Autodesk Inventor part; units mm, degrees
ref_plane "YZ Plane" through (0, 0, 0) normal (1, 0, 0) x (0, 1, 0)
ref_plane "XZ Plane" through (0, 0, 0) normal (0, 1, 0) x (-1, 0, 0)
ref_plane "XY Plane" through (0, 0, 0) normal (0, 0, 1) x (1, 0, 0)
sketch "Esquisse1" plane through (0, 0, 0) normal (0, 0, 1) x (1, 0, 0)
  line L0 (0, -2.6) -> (0, 15.6)
  line L1 (-12.6, 0) -> (5.6, 0)
  line L2 (-10, 10) -> (0, 10)
  line L3 (0, 10) -> (0, 0)
  line L4 (0, 0) -> (-10, 0)
  line L5 (-10, 0) -> (-10, 10)
  line L6 (-10, 10) -> (0, 10)
  line L7 (0, 10) -> (0, 13)
  line L8 (0, 13) -> (-10, 13)
  line L9 (-10, 13) -> (-10, 10)
  line L10 (0, 0) -> (3, 0)
  line L11 (3, 0) -> (3, 13)
  line L12 (3, 13) -> (0, 13)
  line L13 (0, 13) -> (0, 0)
  dimension "d0" = 10
  dimension "d1" = 10
  dimension "d2" = 3
  dimension "d3" = 3
extrude "Extrusion1" add sketch "Esquisse1" along normal blind 2
sketch "Esquisse2" plane through (0, 0, 2) normal (0, 0, 1) x (1, 0, 0)
  line L0 (3, 13) -> (-10, 13)
  line L1 (3, 0) -> (3, 13)
  line L2 (-10, 13) -> (3, 13)
  line L3 (3, 13) -> (3, 10)
  line L4 (3, 10) -> (-10, 10)
  line L5 (-10, 10) -> (-10, 13)
  line L6 (3, 0) -> (0, 0)
  line L7 (0, 0) -> (0, 10)
  line L8 (0, 10) -> (3, 10)
  line L9 (3, 10) -> (3, 0)
  dimension "d6" = 3
  dimension "d7" = 3
extrude "Extrusion2" add sketch "Esquisse2" along normal blind 5
fillet "Congé1" radius 2 1 edges at (3, 13, 3.5)
properties part number "pièce_intérieur_coque_RPI"
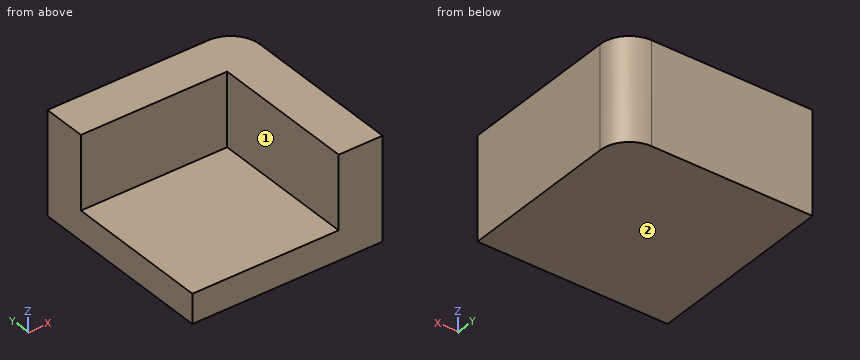
Could you check a few things on this model? Use its own coordinates, in mm. Face numbers are marked on the shaded views. A direction names the side the tool comes from. Give positions to 0.01 mm unless a question says otherwise; leave off trailing zeros. Write each loop counter-clockwise with the first axis right and the second up, starting at its lowest first coordinate (ties: lowest second). Pieces come first, ordered by that corner, then holes. Notation, with made-up numbers: (-29.5, -32) - (-14.5, -32) arc R17 cw to (-14.5, -12) - close; hole circle Ø11 at (-14.5, 86). An arc over 180 degrees is marked (long way). Use CSV: the item, a comma, the result in double quotes. Start each with the question number.
Item 1: For the marked faces 1 and 2, which set-ups out of +Z, -Z, +X, -X, +Y, -Y let a thin tool reach every point of the face, with its end or its side?
Item 2: If I drill on line 1 along Y through (x, z) = (-8.5, 4.25); line 2 along Z through (x, y) = (-7.75, 1); line 3 along X through (y, z) = (9.75, 4.5), over which ranges is the centre line in solid material (lowest first)?
Item 3: I want a section at D-D, the plane y = 12. Please give me the cut outline in (x, z).
Item 4: I'm going to push a flat-ended pin straight in: pin 1 (2.5 mm diameter, centred on x = -3.5, z = 5.5, fed in from -Y). Where does the tip first touch, or does it pass through?
Item 5: I want a section at A-A, the plane z = 6. Please give me the cut outline in (x, y), then the cut area to 3 significant figures.
Item 6: I want a section at C-C, the plane x = -8. Please give me the cut outline in (y, z).
Item 7: I want a section at B-B, the plane y = 7.5. Please give me the cut outline in (x, z), then the cut area to 3 significant figures.
Findings:
1,face 1,"+Z, -X, -Y"
1,face 2,"-Z, +X, -X, +Y, -Y"
2,line 1,"y = 10 to 13"
2,line 2,"z = 0 to 2"
2,line 3,"x = 0 to 3"
3,outline,"(-10, 0) - (2.73, 0) - (2.73, 7) - (-10, 7) - close"
4,pin 1,"stops at y = 10"
5,outline,"(-10, 10) - (0, 10) - (0, 0) - (3, 0) - (3, 11) arc R2 ccw to (1, 13) - (-10, 13) - close"
5,area,"68.1 mm2"
6,outline,"(0, 0) - (13, 0) - (13, 7) - (10, 7) - (10, 2) - (0, 2) - close"
7,outline,"(-10, 0) - (3, 0) - (3, 7) - (0, 7) - (0, 2) - (-10, 2) - close"
7,area,"41.0 mm2"
